from build123d import *

# Parameters (mm, degrees)
F1_DEPTH     = 25.4
F2_W         = 63.5
F2_H         = 38.1
F3_DEPTH     = 12.7
F4_T1_DEPTH  = 63.5
F4_T3_DEPTH  = 38.1
F4_T5_DEPTH  = 50.8
F4_T8_ANGLE  = 180
F4_T10_ANGLE = 180
F4_T15_DEPTH = 76.5641495789
F4_S16_R     = 25.4
F4_T17_DEPTH = 40
F4_T21_DEPTH = 51.1641495789
F4_S22_R     = 25.4
F4_T23_DEPTH = 27
F4_T30_DEPTH = 76.5641495789
F4_S31_R     = 25.4
F4_T32_DEPTH = 40
F4_T36_DEPTH = 51.1641495789
F4_S37_R     = 25.4
F4_T38_DEPTH = 27
F4_T45_DEPTH = 51.1641495789
F4_S46_R     = 25.4
F4_T47_DEPTH = 27
F4_T51_DEPTH = 76.5641495789
F4_S52_R     = 25.4
F4_T53_DEPTH = 40
F4_T60_DEPTH = 76.5641495789
F4_S61_R     = 25.4
F4_T62_DEPTH = 40
F4_T66_DEPTH = 51.1641495789
F4_S67_R     = 25.4
F4_T68_DEPTH = 27
F5_W         = 6.35
F5_H         = 6.35
F5_W_2       = 5.9358693383
F5_H_2       = 6.4880426841
F5_W_3       = 5.79782274
F5_H_3       = 5.521739329
F5_W_4       = 5.9358680336
F5_H_4       = 6.6260866729
F6_DEPTH     = 25.4


# Not quite as in the source:
# - a fillet or chamfer that OpenCascade refuses, or shapes differently, is made with other operations: its cross-section is extruded or revolved along the edge and cut away or added


with BuildPart() as f1:
    # F0 (on Front) → F1 (new body)
    with BuildSketch(Plane.XZ):
        with BuildLine():
            ThreePointArc((-50.8, 0), (-43.3605122421, -17.9605122421), (-25.4, -25.4))
            Line((-25.4, -25.4), (25.4, -25.4))
            ThreePointArc((25.4, -25.4), (43.3605122421, -17.9605122421), (50.8, 0))
            ThreePointArc((50.8, 0), (43.3605122421, 17.9605122421), (25.4, 25.4))
            Line((25.4, 25.4), (-25.4, 25.4))
            ThreePointArc((-25.4, 25.4), (-43.3605122421, 17.9605122421), (-50.8, 0))
        make_face()
    extrude(amount=F1_DEPTH)

    # F2 (on Front) → F3 (cut)
    with BuildSketch(Plane.XZ):
        Rectangle(F2_W, F2_H)
    extrude(amount=F3_DEPTH, mode=Mode.SUBTRACT)

    # F4: chamfer of 5.08 on 8 edges, made by hand

    # F4_s2 → F4_t1 (cut)
    with BuildSketch(Plane.YZ.offset(-31.75)):
        Polygon((0, 24.13), (-5.08, 19.05), (0, 19.05), align=None)
        Polygon((0, -24.13), (-5.08, -19.05), (0, -19.05), align=None)
    extrude(amount=F4_T1_DEPTH, mode=Mode.SUBTRACT)

    # F4_s4 → F4_t3 (cut)
    with BuildSketch(Plane.XY.offset(-19.05)):
        Polygon((-36.83, 0), (-31.75, -5.08), (-31.75, 0), align=None)
        Polygon((36.83, 0), (31.75, -5.08), (31.75, 0), align=None)
    extrude(amount=F4_T3_DEPTH, mode=Mode.SUBTRACT)

    # F4_s6 → F4_t5 (cut)
    with BuildSketch(Plane.YZ.offset(-25.4)):
        Polygon((-20.32, 25.4), (-25.4, 20.32), (-25.4, 25.4), align=None)
        Polygon((-25.4, -20.32), (-20.32, -25.4), (-25.4, -25.4), align=None)
    extrude(amount=F4_T5_DEPTH, mode=Mode.SUBTRACT)

    # F4_s7 → F4_t8 (revolve, cut)
    with BuildSketch(Plane.YZ.offset(-25.4)):
        Polygon((-20.32, -25.4), (-25.4, -20.32), (-25.4, -25.4), align=None)
    revolve(axis=Axis((-25.4, -25.4, 0), (0, 1, 0)), revolution_arc=F4_T8_ANGLE, mode=Mode.SUBTRACT)

    # F4_s9 → F4_t10 (revolve, cut)
    with BuildSketch(Plane.YZ.offset(25.4)):
        Polygon((-25.4, 20.32), (-20.32, 25.4), (-25.4, 25.4), align=None)
    revolve(axis=Axis((25.4, -25.4, 0), (0, 1, 0)), revolution_arc=F4_T10_ANGLE, mode=Mode.SUBTRACT)


with BuildPart() as f4_tool13:
    # F4_s14 → F4_t15 (new body)
    with BuildSketch(Plane.YZ.offset(44.8141495789)):
        Polygon((0, 24.13), (-5.08, 19.05), (0, 19.05), align=None)
    extrude(amount=-F4_T15_DEPTH)

    # F4_s16 → F4_t17 (intersect, symmetric)
    with BuildSketch(Plane.XZ.offset(2.5)):
        with Locations((25.4, 0)):
            Circle(F4_S16_R)
    extrude(amount=F4_T17_DEPTH, both=True, mode=Mode.INTERSECT)

    split(bisect_by=Plane.YZ.offset(31.75), keep=Keep.TOP)


with BuildPart() as f4_tool19:
    # F4_s20 → F4_t21 (new body)
    with BuildSketch(Plane.XY.offset(-19.05)):
        Polygon((36.83, 0), (31.75, -5.08), (31.75, 0), align=None)
    extrude(amount=F4_T21_DEPTH)

    # F4_s22 → F4_t23 (intersect, symmetric)
    with BuildSketch(Plane.XZ.offset(2.5)):
        with Locations((25.4, 0)):
            Circle(F4_S22_R)
    extrude(amount=F4_T23_DEPTH, both=True, mode=Mode.INTERSECT)

    split(bisect_by=Plane.XY.offset(19.05), keep=Keep.TOP)


with BuildPart() as f4_tool13_1:
    add(f4_tool13.part)

    # F4_t25: intersect F4_tool19
    add(f4_tool19.part, mode=Mode.INTERSECT)


with BuildPart() as f1_1:
    add(f1.part)

    # F4_t11: cut F4_tool13
    add(f4_tool13_1.part, mode=Mode.SUBTRACT)


with BuildPart() as f4_tool28:
    # F4_s29 → F4_t30 (new body)
    with BuildSketch(Plane.YZ.offset(31.75)):
        Polygon((0, 24.13), (-5.08, 19.05), (0, 19.05), align=None)
    extrude(amount=-F4_T30_DEPTH)

    # F4_s31 → F4_t32 (intersect, symmetric)
    with BuildSketch(Plane.XZ.offset(2.5)):
        with Locations((-25.4, 0)):
            Circle(F4_S31_R)
    extrude(amount=F4_T32_DEPTH, both=True, mode=Mode.INTERSECT)

    split(bisect_by=Plane.YZ.offset(-31.75), keep=Keep.BOTTOM)


with BuildPart() as f4_tool34:
    # F4_s35 → F4_t36 (new body)
    with BuildSketch(Plane.XY.offset(32.1141495789)):
        Polygon((-36.83, 0), (-31.75, -5.08), (-31.75, 0), align=None)
    extrude(amount=-F4_T36_DEPTH)

    # F4_s37 → F4_t38 (intersect, symmetric)
    with BuildSketch(Plane.XZ.offset(2.5)):
        with Locations((-25.4, 0)):
            Circle(F4_S37_R)
    extrude(amount=F4_T38_DEPTH, both=True, mode=Mode.INTERSECT)

    split(bisect_by=Plane.XY.offset(19.05), keep=Keep.TOP)


with BuildPart() as f4_tool28_1:
    add(f4_tool28.part)

    # F4_t40: intersect F4_tool34
    add(f4_tool34.part, mode=Mode.INTERSECT)


with BuildPart() as f1_2:
    add(f1_1.part)

    # F4_t26: cut F4_tool28
    add(f4_tool28_1.part, mode=Mode.SUBTRACT)


with BuildPart() as f4_tool43:
    # F4_s44 → F4_t45 (new body)
    with BuildSketch(Plane.XY.offset(19.05)):
        Polygon((-36.83, 0), (-31.75, -5.08), (-31.75, 0), align=None)
    extrude(amount=-F4_T45_DEPTH)

    # F4_s46 → F4_t47 (intersect, symmetric)
    with BuildSketch(Plane.XZ.offset(2.5)):
        with Locations((-25.4, 0)):
            Circle(F4_S46_R)
    extrude(amount=F4_T47_DEPTH, both=True, mode=Mode.INTERSECT)

    split(bisect_by=Plane.XY.offset(-19.05), keep=Keep.BOTTOM)


with BuildPart() as f4_tool49:
    # F4_s50 → F4_t51 (new body)
    with BuildSketch(Plane.YZ.offset(-44.8141495789)):
        Polygon((0, -24.13), (-5.08, -19.05), (0, -19.05), align=None)
    extrude(amount=F4_T51_DEPTH)

    # F4_s52 → F4_t53 (intersect, symmetric)
    with BuildSketch(Plane.XZ.offset(2.5)):
        with Locations((-25.4, 0)):
            Circle(F4_S52_R)
    extrude(amount=F4_T53_DEPTH, both=True, mode=Mode.INTERSECT)

    split(bisect_by=Plane.YZ.offset(-31.75), keep=Keep.BOTTOM)


with BuildPart() as f4_tool43_1:
    add(f4_tool43.part)

    # F4_t55: intersect F4_tool49
    add(f4_tool49.part, mode=Mode.INTERSECT)


with BuildPart() as f1_3:
    add(f1_2.part)

    # F4_t41: cut F4_tool43
    add(f4_tool43_1.part, mode=Mode.SUBTRACT)


with BuildPart() as f4_tool58:
    # F4_s59 → F4_t60 (new body)
    with BuildSketch(Plane.YZ.offset(-31.75)):
        Polygon((0, -24.13), (-5.08, -19.05), (0, -19.05), align=None)
    extrude(amount=F4_T60_DEPTH)

    # F4_s61 → F4_t62 (intersect, symmetric)
    with BuildSketch(Plane.XZ.offset(2.5)):
        with Locations((25.4, 0)):
            Circle(F4_S61_R)
    extrude(amount=F4_T62_DEPTH, both=True, mode=Mode.INTERSECT)

    split(bisect_by=Plane.YZ.offset(31.75), keep=Keep.TOP)


with BuildPart() as f4_tool64:
    # F4_s65 → F4_t66 (new body)
    with BuildSketch(Plane.XY.offset(-32.1141495789)):
        Polygon((36.83, 0), (31.75, -5.08), (31.75, 0), align=None)
    extrude(amount=F4_T66_DEPTH)

    # F4_s67 → F4_t68 (intersect, symmetric)
    with BuildSketch(Plane.XZ.offset(2.5)):
        with Locations((25.4, 0)):
            Circle(F4_S67_R)
    extrude(amount=F4_T68_DEPTH, both=True, mode=Mode.INTERSECT)

    split(bisect_by=Plane.XY.offset(-19.05), keep=Keep.BOTTOM)


with BuildPart() as f4_tool58_1:
    add(f4_tool58.part)

    # F4_t70: intersect F4_tool64
    add(f4_tool64.part, mode=Mode.INTERSECT)


with BuildPart() as f1_4:
    add(f1_3.part)

    # F4_t56: cut F4_tool58
    add(f4_tool58_1.part, mode=Mode.SUBTRACT)

    # F5 (on Front) → F6 (join, symmetric)
    with BuildSketch(Plane.XZ):
        with Locations((19.4146236851, 9.9391293569)):
            Rectangle(F5_W, F5_H)
        with Locations((19.2075583543, -10.1461946878)):
            Rectangle(F5_W_2, F5_H_2)
        with Locations((-18.9614597259, -10.3532596925)):
            Rectangle(F5_W_3, F5_H_3)
        with Locations((-19.0304823727, 10.0771726934)):
            Rectangle(F5_W_4, F5_H_4)
    extrude(amount=F6_DEPTH, both=True)


solid = f1_4.part
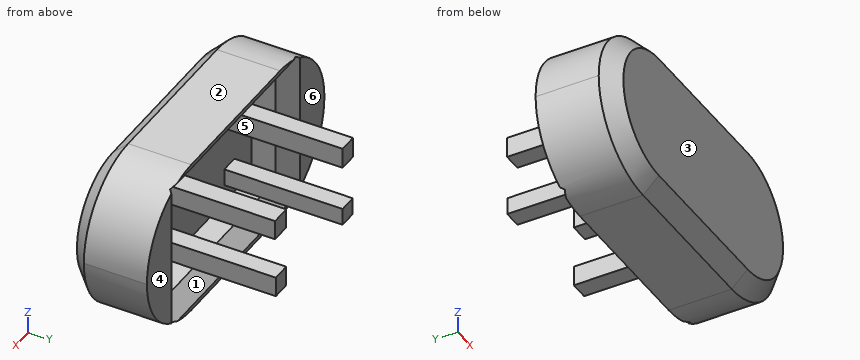
Geometry check sheet. Reference: the model listing, model coordinates, mm. Face numbers are marked on the shaded views. A direction names the side the tool comes from. Round coordinates to 2 decimals unless told otherwise and drop trailing zeros. Write each loop counter-clockwise with the first axis right and the second up, starting at its lowest first coordinate (ties: lowest second). Pieces come first, ordered by that corner, then holes. Notation, with made-up numbers: (31.5, -22.75) - (64.5, -22.75) arc R13 cw to (64.5, -16.75) - close; hole circle Ø5 at (88.25, 29). An arc over 180 degrees is marked (long way). One line per item, written item: value.
1. Cross-section at A-A on y = -7. Record the boundary of the cut face in (x, z).
The answers:
outline: (-25.4, -25.4) - (25.4, -25.4) arc R25.4 ccw to (25.4, 25.4) - (-25.4, 25.4) arc R25.4 ccw to start; (-22, 6.76) - (-16.06, 6.76) - (-16.06, 13.39) - (-22, 13.39) - close; (-21.86, -13.11) - (-16.06, -13.11) - (-16.06, -7.59) - (-21.86, -7.59) - close; (16.24, -13.39) - (22.18, -13.39) - (22.18, -6.9) - (16.24, -6.9) - close; (16.24, 6.76) - (22.59, 6.76) - (22.59, 13.11) - (16.24, 13.11) - close; hole (-31.75, -19.05) - (31.75, -19.05) - (31.75, 19.05) - (-31.75, 19.05) - close
2. Scan lines: L1, parallel to Z at x = 18, y = 15.5; L2, parallel to Z at x = 3, y = -7; L3, parallel to X at y = -12.5, z = -11.5. Record each from-to range of solid material in increasing order.
The answers:
L1: z = -13.39 to -6.9, 6.76 to 13.11
L2: z = -25.4 to -19.05, 19.05 to 25.4
L3: x = -48.05 to -31.75, -21.86 to -16.06, 16.24 to 22.18, 31.75 to 48.05
3. Cross-section at C-C on y = 21.5. Record the boundary of the cut face in (x, z), and give its area (3 significant figures).
The answers:
outline: (-22, 6.76) - (-16.06, 6.76) - (-16.06, 13.39) - (-22, 13.39) - close; (-21.86, -13.11) - (-16.06, -13.11) - (-16.06, -7.59) - (-21.86, -7.59) - close; (16.24, -13.39) - (22.18, -13.39) - (22.18, -6.9) - (16.24, -6.9) - close; (16.24, 6.76) - (22.59, 6.76) - (22.59, 13.11) - (16.24, 13.11) - close
area: 150 mm^2
4. Cross-section at D-D on y = -17.5. Record the boundary of the cut face in (x, z), and give its area (3 significant figures).
The answers:
outline: (-25.4, -25.4) - (25.4, -25.4) arc R25.4 ccw to (25.4, 25.4) - (-25.4, 25.4) arc R25.4 ccw to start
area: 4,610 mm^2
5. Set-up check for the marked faces 4, 5 and 6: record each of +Z, -Z, +X, -X, +Y, -Y from which the full face is reachable in a straight line by a thin tool's end or side.
The answers:
face 4: +Z, -Z, +X, +Y
face 5: +Y
face 6: +Z, -Z, -X, +Y
6. Mould release check, pull along Z, two halves, no side actions. Record for the marked faces 1, 2 and 3: released by +Z, released by -Z, zero draft, split by the parting line, or undercut.
The answers:
face 1: undercut
face 2: released by +Z
face 3: zero draft
7. Cross-section at B-B on x = 8. Record the boundary of the cut face in (y, z), and give its area (3 significant figures).
The answers:
outline: (-25.4, -20.32) - (-20.32, -25.4) - (0, -25.4) - (0, -24.13) - (-5.08, -19.05) - (-12.7, -19.05) - (-12.7, 19.05) - (-5.08, 19.05) - (0, 24.13) - (0, 25.4) - (-20.32, 25.4) - (-25.4, 20.32) - close
area: 755 mm^2
8. Depth check by flat-ended pin: pin 1 Ø8.5 at (y, z) = (-10, 2) entering from -X; pin 2 Ø6 at (x, z) = (-10.5, -1.5) entering from +Y; pin 3 Ø5 at (y, z) = (4, -9.5) entering from +X; pin 4 Ø7 at (x, z) = (42.5, 10.5) entering from +Y. Enter the tip coordinate at first touch or a pass-through.
The answers:
pin 1: stops at x = -50.8
pin 2: stops at y = -12.7
pin 3: stops at x = 22.18
pin 4: stops at y = 0
